from build123d import *

# Parameters (mm, degrees)
M12_TAPPED_HOLE1_D      = 10.2
M12_TAPPED_HOLE1_DEPTH  = 35
M12_TAPPED_HOLE1_TIP    = 3.064389157
CUT_EXTRUDE1_DEPTH      = 245.361412666
CUT_EXTRUDE1_DEPTH_BACK = 245.361412666
SKETCH4_R               = 6
CHAMFER1_SIZE           = 1


with BuildPart() as part:
    # Sketch1 → Revolve1 (revolve)
    with BuildSketch(Plane.XY, mode=Mode.PRIVATE) as revolve1_sk:
        Polygon((0, 0), (0, 240), (11, 240), (11, 227), (22.5, 227), (32.5, 217), (32.5, 167), (22.5, 157), (19, 157), (19, 0), align=None)
    revolve(revolve1_sk.sketch.rotate(Axis((0, 0, 0), (0, 1, 0)), 90), axis=Axis((0, 0, 0), (0, 1, 0)))

    # M12 Tapped Hole1
    with Locations(Plane.ZX.offset(240)):
        with Locations((0, 0)):
            Hole(M12_TAPPED_HOLE1_D / 2, depth=M12_TAPPED_HOLE1_DEPTH)
            with Locations((0, 0, -(M12_TAPPED_HOLE1_DEPTH + M12_TAPPED_HOLE1_TIP / 2))):  # 118° drill point
                Cone(0, M12_TAPPED_HOLE1_D / 2, M12_TAPPED_HOLE1_TIP, mode=Mode.SUBTRACT)

    # Sketch4 → Cut-Extrude1 (cut, two sides: drawn at the far end of the back side and taken through both)
    with BuildSketch(Plane.XY.offset(-CUT_EXTRUDE1_DEPTH_BACK)):
        with Locations((0, 192)):
            Circle(SKETCH4_R)
    extrude(amount=CUT_EXTRUDE1_DEPTH + CUT_EXTRUDE1_DEPTH_BACK, mode=Mode.SUBTRACT)

    # Chamfer1
    chamfer1_edges = [part.edges().sort_by_distance(p)[0] for p in [
        (0, 240, 5.1),
    ]]
    chamfer(chamfer1_edges, length=CHAMFER1_SIZE)


solid = part.part
CAD build for the part. Positions are in the model's coordinates, mm. A direction names the side the tool comes from. Round coordinates to 2 decimals unless told otherwise and drop trailing zeros. Write each loop counter-clockwise with the first axis right and the second up, starting at its lowest first coordinate (ties: lowest second). Pieces come first, ordered by that corner, then holes. Notation, with made-up numbers: M 61.5,26 L 115.5,26 A22 cw 115.5,56 Z; hole C -15,60 d10. An arc over 180 degrees is marked long. Use a Markdown table: item, result. Add a question column.
1. Drill centre lines: probe 1 along X at (y, z) = (192, 0); probe 2 along Y at (x, z) = (0, -1); probe 3 along Z at (x, y) = (-0.5, 76). Where is each one in solid material? Low to high.
2. Slice it at A-A on y = 169.5. Give the cut face in (x, z), then the cut area to 3 significant figures.
3. Flat gauge pins, fed straight in: P1, Ø4, axis at y = 89, z = 1, coming from the -X side; P2, Ø2, axis at y = 37, z = -21, coming from the +X side; P3, Ø1, axis at x = 20.5, z = 11, coming from the +Y side; P4, Ø10, axis at x = 26, z = 23.5, coming from the -Y side. Where does each tip first touch, or does it go through?
4. Pull direction Z, two halves, no side cores. Call faces 1 (the face through (-0.865, 202.468, -0.192)), 2 (the face through (-4.5, 221.8, -2.4)), 3 (the face through (10.74, 233.41, 2.38)), 4 (the face through (10, 227, -5)): released by +Z, released by -Z, zero draft, split by the parting line, or undercut.
5. 3-axis set-ups, long thin cutter, end or side, ignore diameter. For faces 5 (the face through (-9.76, 191.65, -31)), 6 (the face through (18.548, 77.401, 4.119)): which of +Z, -Z, +X, -X, +Y, -Y reach the whole face in a straight line?
Reply:
| question | item | result |
|---|---|---|
| 1 | probe 1 | x = -32.5 to -6, 6 to 32.5 |
| 1 | probe 2 | y = 0 to 186, 198 to 202.54 |
| 1 | probe 3 | z = -18.99 to 18.99 |
| 2 | outline | C 0,0 d65 |
| 2 | area | 3,320 mm^2 |
| 3 | P1 | stops at x = -19 |
| 3 | P2 | passes through |
| 3 | P3 | stops at y = 226.74 |
| 3 | P4 | stops at y = 164.55 |
| 4 | face 1 | undercut |
| 4 | face 2 | undercut |
| 4 | face 3 | split by the parting line |
| 4 | face 4 | zero draft |
| 5 | face 5 | +Y, -Y |
| 5 | face 6 | -Y |
